Autodesk Inventor part; units mm, degrees
ref_plane "YZ Plane" through (0, 0, 0) normal (1, 0, 0) x (0, 1, 0)
ref_plane "XZ Plane" through (0, 0, 0) normal (0, 1, 0) x (-1, 0, 0)
ref_plane "XY Plane" through (0, 0, 0) normal (0, 0, 1) x (1, 0, 0)
sketch "Sketch1" plane through (0, 0, 0) normal (0, 1, 0) x (-1, 0, 0)
  line L0 (20, -20) -> (-20, -20)
  line L1 (-20, -20) -> (-20, 20)
  line L2 (-20, 20) -> (20, 20)
  line L3 (20, 20) -> (20, -20)
  line L4 (20, -20) -> (-20, 20) construction
  line L5 (-20, -20) -> (20, 20) construction
  point P0 (0, 0)
  dimension "d0" = 40
  dimension "d1" = 40
extrude "Extrusion1" add sketch "Sketch1" along normal blind 7
sketch "Sketch2" plane through (0, 7, 0) normal (0, 1, 0) x (1, 0, 0)
  line L0 (-20, -20) -> (20, -20)
  point P0 (0, 0)
  point P1 (0, -10)
  point P2 (0, 10)
  dimension "d4" = 20
  dimension "d5" = 10
sketch "Sketch3" plane through (20, 0, -20) normal (0, 0, -1) x (-1, 0, 0)
  line L0 (0, 0) -> (0, 7)
  line L1 (0, 0) -> (40, 0)
  line L2 (40, 0) -> (40, 50)
  line L3 (40, 50) -> (0, 50)
  line L4 (0, 50) -> (0, 0)
  point P0 (20, 0)
  dimension "d14" = 50
  dimension "d15" = 40
extrude "Extrusion2" add sketch "Sketch3" along normal blind 7
fillet "Fillet2" radius 3 1 edges at (0, 7, -20)
fillet "Fillet2" radius 5 4 edges at (-20, 50, -23.5) (20, 50, -23.5) (-20, 3.5, 20) (20, 3.5, 20)
fillet "Fillet2" radius 2 1 edges at (0, 0, -27)
sketch "Sketch4" plane through (20, 0, -20) normal (0, 0, 1) x (1, 0, 0)
  line L0 (-35, 0) -> (-5, 0)
  line L1 (-40, 7) -> (0, 7)
  point P0 (-20, 0)
  point P1 (-20, 39.5)
  point P2 (-20, 19.5)
  point P3 (-20, 0)
  point P4 (-20, 0)
  dimension "d22" = 20
  dimension "d23" = 12.5
hole "Hole4" at (0, 39.5, -20) at (0, 19.5, -20) direction (0, 0, -1) diameter 5.4 end through all
hole "Hole5" at (0, 7, 10) at (0, 7, -10) direction (0, -1, 0) diameter 5.4 end through all
properties part number "angulares"
Can you work these out from the model? Positions are in its coordinate system, mm. A direction names the side the tool comes from. Coordinates: 2 decimals unless noted, no trailing zeros. Write each loop counter-clockwise with the first axis right and the second up, starting at its lowest first coordinate (ties: lowest second). Pieces come first, ordered by that corner, then holes. Notation, with made-up numbers: M -35,76.5 L -24,76.5 A12 cw -24,86.5 Z; hole C -20,-38.75 d4. An arc over 180 degrees is marked long. Use one line per item in the form item = value.
Q1. If we section it at C-C (y = 39.5): Write out the boundary of the cut face in (x, z).
Model answer:
outline = M -20,-27 L -2.7,-27 L -2.7,-20 L -20,-20 Z; M 2.7,-27 L 20,-27 L 20,-20 L 2.7,-20 Z
Q2. For P1, Ø3, axis at x = 0, z = 10, coming from the +Y side; P2, Ø1.5, axis at x = 15, z = -12, coming from the +Y side, each with a flat end and sliding along its axis, tell me the tip position at first contact or that it passes through.
Model answer:
P1 = through
P2 = 7
Q3. I need wall thicknesses on line 1 along Z through (x, y) = (0, 2); line 2 along X through (y, z) = (5, -10); line 3 along Z through (x, y) = (18.5, 38). Which ranges of each line are inside material? Lowest first, please. Write a range as from..to.
Model answer:
line_1 = -27..-12.7, -7.3..7.3, 12.7..20
line_2 = -20..-2.7, 2.7..20
line_3 = -27..-20
Q4. If we section it at A-A (x = 0): Write out the boundary of the cut face in (y, z), then the cut area to 3 significant figures.
Model answer:
outline = M 0,-25 A2 ccw 2,-27 L 16.8,-27 L 16.8,-20 L 10,-20 A3 cw 7,-17 L 7,-12.7 L 0,-12.7 Z; M 0,-7.3 L 7,-7.3 L 7,7.3 L 0,7.3 Z; M 0,12.7 L 7,12.7 L 7,20 L 0,20 Z; M 22.2,-27 L 36.8,-27 L 36.8,-20 L 22.2,-20 Z; M 42.2,-27 L 50,-27 L 50,-20 L 42.2,-20 Z
area = 480 mm^2
Q5. We'd pull the mould along Y, two halves only. Please class faces 1 (the cylindrical face through (-19, 48, -24)), 2 (the cylindrical face through (1.034, 17.006, -23.549)), 3 (the cylindrical face through (18, 4, 19)): +Y half, -Y half, draft (parallel to the pull), parting line (faces both ways), or undercut.
Model answer:
face_1 = +Y half
face_2 = undercut
face_3 = draft
Q6. If we section it at B-B (z = -23): Write out the boundary of the cut face in (x, y), then the cut area to 3 significant figures.
Model answer:
outline = M -20,0 L 20,0 L 20,45 A5 ccw 15,50 L -15,50 A5 ccw -20,45 Z; hole C 0,19.5 d5.4; hole C 0,39.5 d5.4
area = 1,940 mm^2
Q7. If we section it at D-D (z = -10): Write out the boundary of the cut face in (x, y), then the cut area to 3 significant figures.
Model answer:
outline = M -20,0 L -2.7,0 L -2.7,7 L -20,7 Z; M 2.7,0 L 20,0 L 20,7 L 2.7,7 Z
area = 242 mm^2
Q8. For faces 4 (the flat face through (0, 50, -23)), 5 (the flat face through (0, 30, -20)), which set-ups out of +Z, -Z, +X, -X, +Y, -Y let a thin tool reach every point of the face, with its end or its side?
Model answer:
face_4 = +Z, -Z, +X, -X, +Y
face_5 = +Z, +X, -X, +Y
